Geometry: see drawing. Coordinates: mm, zero at the bounding-box minimum. A direction names the side the tool comes from. Give positions to 0.01 mm unless a question says otherwise; leave off trailing zeros. Order: outer loops, then holes, each group sorted by start corner. A loop starts at its lowest first (then second) coordinate and runs counter-clockwise, first axis right, second up. Notation, with made-up numbers: M 21.5,-13.5 L 37.5,-13.5 A20 cw 37.5,-4.5 Z; hole C -22.5,76 d4. An arc over 180 degrees is marked long. Answer as a JSON object with one key per item and string values. Group by question number.
1. Section query A-A (x = 10). Output: boundary loops of the cut face in (y, z).
2. Section query B-B (x = 18.5). Output: boundary loops of the cut face in (y, z), plus the area to 3 significant figures.
3. Set-up query: the marked faces 1 and 2. Return all of +Z, -Z, +X, -X, +Y, -Y with unobstructed straight access to the full face (end or side cutting, diameter ignored); none if empty.
4. Section query C-C (z = 46). Output: boundary loops of the cut face in (x, y).
5. Material intervals for L1, parallel to Z at x = 11, y = 32.5; L2, parallel to Y at x = 64, z = 59; L3, parallel to Y at x = 35, z = 71.15 (1 decimal), sorted ascending. Write a range as [from, to].
6. Section query D-D (y = 34). Output: boundary loops of the cut face in (x, z).
7. Pin query (flat end, axial travel): P1, Ø2, axis at x = 17, y = 15.5, coming from the -Z side; P2, Ø6, axis at x = 20, z = 39, coming from the -Y side; P3, Ø7.5, axis at x = 10, y = 18.39, coming from the +Z side. Return the tip coordinate at first contact, or that it passes through.
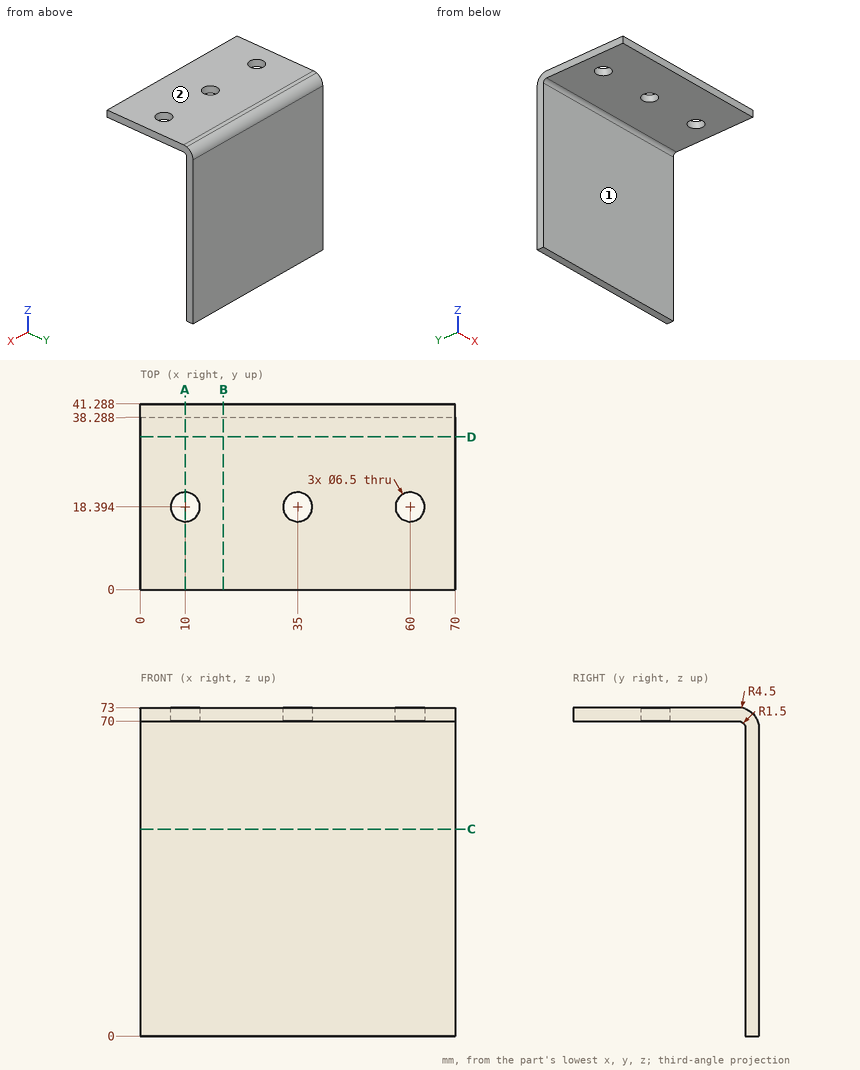
Answer sheet:
{
 "1": {"outline": "M 0,70 L 15.14,70 L 15.14,73 L 0,73 Z; M 21.64,70 L 36.79,70 A1.5 cw 38.29,68.5 L 38.29,0 L 41.29,0 L 41.29,68.5 A4.5 ccw 36.79,73 L 21.64,73 Z"},
 "2": {"outline": "M 0,70 L 36.79,70 A1.5 cw 38.29,68.5 L 38.29,0 L 41.29,0 L 41.29,68.5 A4.5 ccw 36.79,73 L 0,73 Z", "area": "330 mm^2"},
 "3": {"face 1": "-Z, +X, -X, -Y", "face 2": "+Z, +X, -X, +Y, -Y"},
 "4": {"outline": "M 0,38.29 L 70,38.29 L 70,41.29 L 0,41.29 Z"},
 "5": {"L1": "[70, 73]", "L2": "[38.29, 41.29]", "L3": "[0, 15.1], [21.6, 40.4]"},
 "6": {"outline": "M 0,70 L 70,70 L 70,73 L 0,73 Z"},
 "7": {"P1": "z = 70", "P2": "y = 38.29", "P3": "z = 73"}
}
